Could you check a few things on this model? Use its own coordinates, in mm. A direction names the side the tool comes from. Coordinates: 2 decimals unless noted, no trailing zeros. Order: outer loops, then holes, each group sorted by start corner. A loop starts at its lowest first (then second) coordinate and runs counter-clockwise, first axis right, second up. Notation, with made-up numbers: (85, 1) -> (111, 1) arc R33 cw to (111, 29) -> close; hole circle Ø2 at (-17.75, 88.25). An arc over 180 degrees is marked (long way). Use a Markdown table: item, result. Add a question column.
1) If we section it at C-C (z = 49): Write out the boundary of the cut face in (x, y) (3 decimals).
2) If we section it at A-A (z = 24): Write out the boundary of the cut face in (x, y) (3 decimals), plus the area to 3 significant figures.
3) If we section it at B-B (x = 51): Write out the boundary of the cut face in (y, z).
4) If I drill on L1, parallel to Y at x = -19, z = 43.5 (3 decimals); L2, parallel to X at y = -12, z = 53.5; L3, parallel to Y at x = 10, z = 18.5 (3 decimals), over which ranges is the centre line in solid material (lowest first)? Write a range as [from, to].
5) If we section it at D-D (x = -41): Write out the boundary of the cut face in (y, z) (3 decimals), plus the area to 3 significant figures.
6) Which directions (+Z, -Z, +X, -X, +Y, -Y) give clear straight access to the entire face, cutting with the end or side of a thin tool? Please do faces 1 (the flat face through (3.009, -12, 46)), 2 (the flat face through (0, -14.753, 49)), 3 (the flat face through (-24, -5, 17.742)), 4 (the flat face through (-18, 6.771, 43)), 5 (the flat face through (-24, -9.601, 11)).
7) Thinking about a two-plate mould opening in Y: for faces 6 (the flat face through (-14.908, -5, 43)), 7 (the flat face through (-49.8, -5, 3)), 8 (the flat face through (-4, -23.205, 35)), which applies, +Y half, -Y half, draft (parallel to the pull), parting line (faces both ways), or undercut?
8) Will these pins go through, and if not, where does the flat tip stop? pin 1 Ø1.6 at (x, y) = (-18.5, -7) entering from +Z; pin 2 Ø6 at (y, z) = (-11, 34.5) entering from -X; pin 3 Ø1 at (y, z) = (2, 19) entering from +X; pin 4 Ø4 at (x, y) = (-33.5, 9.5) entering from -Z.
```python
from build123d import *

# Parameters (mm, degrees)
F0_W      = 99.6
F0_H      = 27.37
F0_R      = 9.265
F1_DEPTH  = 5.32
F2_W      = 37.4
F2_H      = 27.37
F2_R      = 9.265
F3_DEPTH  = 51.95
F5_DEPTH  = 9.52
F7_DEPTH  = 22.25
F10_DEPTH = 37.475
F12_DEPTH = 7.5
F14_DEPTH = 5.25
F15_R     = 0.6044453377
F16_DEPTH = 25
F18_W     = 32.5579583809
F18_H     = 4.8552089012
F19_DEPTH = 52
F21_DEPTH = 4.825
F22_DEPTH = 25


with BuildPart() as f1:
    # F0 (on Top) → F1 (new body)
    with BuildSketch(Plane.XY):
        Rectangle(F0_W, F0_H)
        Circle(F0_R, mode=Mode.SUBTRACT)
    extrude(amount=F1_DEPTH)

    # F2 (on face) → F3 (join)
    with BuildSketch(Plane.XY.offset(5.32)):
        with Locations((-1.4579583809, 0)):
            Rectangle(F2_W, F2_H)
        Circle(F2_R, mode=Mode.SUBTRACT)
    extrude(amount=F3_DEPTH)

    # F4 (on face) → F5 (join)
    with BuildSketch(Plane.XZ.offset(13.685)):
        Polygon((-49.8, 0), (-15.7770887017, 0), (-15.7770887017, 12.8972763196), (0, 41.4250344038), (13.8749163598, 14.3025843427), (13.8749163598, 0), (49.8, 0), (49.8, 5.32), (17.2420416191, 5.32), (17.2420416191, 57.27), (-20.1579583809, 57.27), (-20.1579583809, 5.32), (-49.8, 5.32), align=None)
    extrude(amount=F5_DEPTH)

    # F6 (on face) → F7 (cut)
    with BuildSketch(Plane.XY.offset(57.27)):
        with BuildLine():
            ThreePointArc((3.0086552724, -8.7628887047), (-0.017033567, -9.264984342), (-3.0408557647, -8.7517667484))
            Line((-3.0408557647, -8.7517667484), (-3.0408557647, -14.7527681977))
            Line((-3.0408557647, -14.7527681977), (3.0086552724, -14.7527681977))
            Line((3.0086552724, -14.7527681977), (3.0086552724, -8.7628887047))
        make_face()
    extrude(amount=-F7_DEPTH, mode=Mode.SUBTRACT)

    # F9 (on face) → F10 (cut)
    with BuildSketch(Plane.XZ.offset(23.205)):
        with BuildLine():
            Line((-20.1579583809, 27.9725342989), (-20.1579583809, 17.8241562098))
            ThreePointArc((-20.1579583809, 17.8241562098), (-15.9551803728, 22.8983452544), (-20.1579583809, 27.9725342989))
        make_face()
    extrude(amount=-F10_DEPTH, mode=Mode.SUBTRACT)

    # F11 (on face) → F12 (join)
    with BuildSketch(Plane(origin=(-20.1579583809, 0, 0), x_dir=(0, -1, 0), z_dir=(-1, 0, 0))):
        Polygon((0, 17.7417956293), (0, 5.4170973599), (9.6006197855, 5.3354022093), (9.6006197855, 17.7417956293), align=None)
    extrude(amount=F12_DEPTH)

    # F13 (on face) → F14 (cut)
    with BuildSketch(Plane(origin=(-20.1579583809, 0, 0), x_dir=(0, -1, 0), z_dir=(-1, 0, 0))):
        Polygon((8.0970225025, 57.27), (-6.7709684372, 57.27), (-6.7709684372, 28.0677657574), (16.8139953166, 28.0677657574), (16.8139953166, 57.0610500872), align=None)
    extrude(amount=-F14_DEPTH, mode=Mode.SUBTRACT)

    # F15 (on face) → F16 (cut)
    with BuildSketch(Plane.XZ.offset(9.6006197855)):
        with Locations((-26.3735596091, 15.4167022556)):
            Circle(F15_R)
    extrude(amount=-F16_DEPTH, mode=Mode.SUBTRACT)

    # F18 (on face) → F19 (join)
    with BuildSketch(Plane.XY.offset(5.32)):
        with Locations((33.5210208096, 11.2573955494)):
            Rectangle(F18_W, F18_H)
    extrude(amount=F19_DEPTH)

    # F20 (on face) → F21 (join)
    with BuildSketch(Plane.XZ.offset(-8.8297910988)):
        with BuildLine():
            Line((49.8, 57.32), (49.8, 44.2806235084))
            ThreePointArc((49.8, 44.2806235084), (53.5530649007, 39.3313205539), (54.8859158534, 33.2646407187))
            ThreePointArc((54.8859158534, 33.2646407187), (53.5530649007, 27.1979608835), (49.8, 22.248657929))
            Line((49.8, 22.248657929), (49.8, 5.32))
            Line((49.8, 5.32), (66.4364546537, 29.0281493217))
            ThreePointArc((66.4364546537, 29.0281493217), (67.8548424387, 33.0029604957), (66.4364546537, 36.9777716696))
            Line((66.4364546537, 36.9777716696), (49.8, 57.32))
        make_face()
    extrude(amount=-F21_DEPTH)

    # F20 (on face) → F22 (cut)
    with BuildSketch(Plane.XZ.offset(-8.8297910988)):
        with BuildLine():
            ThreePointArc((25.9396215898, 33.2646407187), (40.4127687216, 18.7914935869), (54.8859158534, 33.2646407187))
            ThreePointArc((54.8859158534, 33.2646407187), (40.4127687216, 47.7377878505), (25.9396215898, 33.2646407187))
        make_face()
    extrude(amount=-F22_DEPTH, mode=Mode.SUBTRACT)


solid = f1.part
```
Answer sheet:
| question | item | result |
|---|---|---|
| 1 | outline | (-20.158, -23.205) -> (17.242, -23.205) -> (17.242, 8.83) -> (56.604, 8.83) -> (56.604, 13.655) -> (49.8, 13.655) -> (49.8, 13.685) -> (-20.158, 13.685) -> (-20.158, 6.771) -> (-14.908, 6.771) -> (-14.908, -16.814) -> (-20.158, -16.814) -> close; hole (-3.041, -14.753) -> (3.009, -14.753) -> (3.009, -8.763) arc R9.265 ccw (long way) to (-3.041, -8.752) -> close |
| 2 | outline | (-16.074, -23.205) -> (-9.637, -23.205) -> (-9.637, -13.685) -> (8.914, -13.685) -> (8.914, -23.205) -> (17.242, -23.205) -> (17.242, 8.83) -> (29.293, 8.83) -> (29.293, 13.685) -> (-16.074, 13.685) -> close; (51.532, 8.83) -> (62.908, 8.83) -> (62.908, 13.655) -> (51.532, 13.655) -> close; hole circle Ø18.53 at (0, 0) |
| 2 | area | 896 mm2 |
| 3 | outline | (8.83, 7.03) -> (13.65, 7.03) -> (13.65, 23.4) -> (8.83, 23.4) -> close; (8.83, 43.13) -> (13.65, 43.13) -> (13.65, 55.85) -> (8.83, 55.85) -> close |
| 4 | L1 | [-23.205, -16.814], [6.771, 13.685] |
| 4 | L2 | [-14.91, -3.04], [3.01, 17.24] |
| 4 | L3 | [-13.685, 13.685] |
| 5 | outline | (-23.205, 0) -> (13.685, 0) -> (13.685, 5.32) -> (-23.205, 5.32) -> close |
| 5 | area | 196 mm2 |
| 6 | face 1 | +Z |
| 6 | face 2 | +Z, -Z |
| 6 | face 3 | +Z, -X, +Y, -Y |
| 6 | face 4 | +Z, -X |
| 6 | face 5 | +Z, -X, -Y |
| 7 | face 6 | undercut |
| 7 | face 7 | draft |
| 7 | face 8 | -Y half |
| 8 | pin 1 | z = 28.07 |
| 8 | pin 2 | x = -14.91 |
| 8 | pin 3 | x = 17.24 |
| 8 | pin 4 | z = 0 |
